Read the model definition and answer for the solid it produces. Units are mm, in the model's axes. Face numbers are marked on the shaded views. A direction names the side the tool comes from. Give positions to 0.01 mm unless a question says otherwise; leave off trailing zeros. Order: outer loops, then holes, each group sorted by start corner. A loop starts at its lowest first (then second) coordinate and runs counter-clockwise, first axis right, second up. Notation, with made-up numbers: (-33, 10) - (-26, 10) arc R32 ccw to (-26, 37) - close; hole circle Ø10 at (-8, -10.75). An arc over 180 degrees is marked (long way). Use a Markdown table: item, result. Add a question column.
1. A cutting plane is placed at D-D on x = 7.5. Determine the outline of the cut face in (y, z).
2. A flat-ended cylindrical pin translates along its axis: P1, Ø1.5, axis at x = -20.5, y = 2.5, coming from the +Z side. Find the tip coordinate at first contact, or state that the pin passes through.
3. A cutting plane is placed at C-C on z = 7.75. Determine the outline of the cut face in (x, y).
4. A cutting plane is placed at A-A on y = 0. Determine the outline of the cut face in (x, z).
5. Which of the six approach directions +Z, -Z, +X, -X, +Y, -Y give full straight-line access (tool end or side, diameter ignored) to the marked faces 1, 2 and 3?
6. A cutting plane is placed at B-B on y = -24.5. Determine the outline of the cut face in (x, z).
7. Consider L1, parallel to X at y = 0, z = 1.5; L2, parallel to X at y = -11, z = 3.75; L3, parallel to Y at x = -2, z = 3.5. Determine where each line is inside the solid, lowest interval first.
8. For a pull along Y with two mould halves and no side action, classify the marked faces 4, 5 and 6 as released by +Y, released by -Y, zero draft, split by the parting line, or undercut.
```python
from build123d import *

# Parameters (mm, degrees)
F0_W     = 56.9
F0_H     = 61.77927
F0_R     = 4.45
F1_DEPTH = 3
F2_R     = 4.45
F4_DEPTH = 10
F5_DEPTH = 3
F6_R     = 1.25
F7_DEPTH = 40


with BuildPart() as f1:
    # F0 (on Top) → F1 (new body)
    with BuildSketch(Plane.XY):
        Rectangle(F0_W, F0_H)
        with BuildLine():
            Line((1.5, -16.92031), (1.5, -26.92031))
            ThreePointArc((1.5, -26.92031), (1.06066, -27.98097), (0, -28.42031))
            ThreePointArc((0, -28.42031), (-1.06066, -27.98097), (-1.5, -26.92031))
            Line((-1.5, -26.92031), (-1.5, -16.92031))
            ThreePointArc((-1.5, -16.92031), (-1.06066, -15.85965), (0, -15.42031))
            ThreePointArc((0, -15.42031), (1.06066, -15.85965), (1.5, -16.92031))
        make_face(mode=Mode.SUBTRACT)
        with BuildLine():
            Line((-23.42031, -3.5), (-23.42031, 0))
            Line((-23.42031, 0), (-23.42031, 3.5))
            ThreePointArc((-23.42031, 3.5), (-21.92031, 5), (-20.42031, 3.5))
            Line((-20.42031, 3.5), (-20.42031, 0))
            Line((-20.42031, 0), (-20.42031, -3.5))
            ThreePointArc((-20.42031, -3.5), (-21.92031, -5), (-23.42031, -3.5))
        make_face(mode=Mode.SUBTRACT)
        with Locations((-20, 12)):
            Circle(F0_R, mode=Mode.SUBTRACT)
        with BuildLine():
            Line((-11.5, -3.5), (-11.5, 0))
            Line((-11.5, 0), (-11.5, 3.5))
            ThreePointArc((-11.5, 3.5), (-8.131728, 11.631728), (0, 15))
            ThreePointArc((0, 15), (8.131728, 11.631728), (11.5, 3.5))
            Line((11.5, 3.5), (11.5, 0))
            Line((11.5, 0), (11.5, -3.5))
            ThreePointArc((11.5, -3.5), (8.131728, -11.631728), (0, -15))
            ThreePointArc((0, -15), (-8.131728, -11.631728), (-11.5, -3.5))
        make_face(mode=Mode.SUBTRACT)
        with BuildLine():
            Line((20.42031, -3.5), (20.42031, 0))
            Line((20.42031, 0), (20.42031, 3.5))
            ThreePointArc((20.42031, 3.5), (21.92031, 5), (23.42031, 3.5))
            Line((23.42031, 3.5), (23.42031, 0))
            Line((23.42031, 0), (23.42031, -3.5))
            ThreePointArc((23.42031, -3.5), (21.92031, -5), (20.42031, -3.5))
        make_face(mode=Mode.SUBTRACT)
        with Locations((20, 12)):
            Circle(F0_R, mode=Mode.SUBTRACT)
        with BuildLine():
            Line((-1.5, 16.92031), (-1.5, 26.92031))
            ThreePointArc((-1.5, 26.92031), (-1.06066, 27.98097), (0, 28.42031))
            ThreePointArc((0, 28.42031), (1.06066, 27.98097), (1.5, 26.92031))
            Line((1.5, 26.92031), (1.5, 16.92031))
            ThreePointArc((1.5, 16.92031), (1.06066, 15.85965), (0, 15.42031))
            ThreePointArc((0, 15.42031), (-1.06066, 15.85965), (-1.5, 16.92031))
        make_face(mode=Mode.SUBTRACT)
    extrude(amount=F1_DEPTH)

    # F2 (on face) → F4 (join)
    with BuildSketch(Plane.XY.offset(3)):
        with BuildLine():
            Line((-26.45, -30.889635), (-26.45, 9.411564))
            ThreePointArc((-26.45, 9.411564), (-13.05, 12), (-26.45, 14.588436))
            Line((-26.45, 14.588436), (-26.45, 28.889635))
            Line((-26.45, 28.889635), (26.45, 28.889635))
            Line((26.45, 28.889635), (26.45, 14.588436))
            ThreePointArc((26.45, 14.588436), (13.05, 12), (26.45, 9.411564))
            Line((26.45, 9.411564), (26.45, -30.889635))
            Line((26.45, -30.889635), (28.45, -30.889635))
            Line((28.45, -30.889635), (28.45, 30.889635))
            Line((28.45, 30.889635), (-28.45, 30.889635))
            Line((-28.45, 30.889635), (-28.45, -30.889635))
            Line((-28.45, -30.889635), (-26.45, -30.889635))
        make_face()
        with Locations((-20, 12)):
            Circle(F2_R, mode=Mode.SUBTRACT)
        with Locations((20, 12)):
            Circle(F2_R, mode=Mode.SUBTRACT)
    extrude(amount=F4_DEPTH)

    # F3 (on face) → F5 (join)
    with BuildSketch(Plane.XY.offset(3)):
        with BuildLine():
            ThreePointArc((-19.42031, 3.5), (-21.92031, 6), (-24.42031, 3.5))
            Line((-24.42031, 3.5), (-24.42031, -3.5))
            ThreePointArc((-24.42031, -3.5), (-21.92031, -6), (-19.42031, -3.5))
            Line((-19.42031, -3.5), (-19.42031, 3.5))
        make_face()
        with BuildLine():
            ThreePointArc((-23.42031, 3.5), (-21.92031, 5), (-20.42031, 3.5))
            Line((-20.42031, 3.5), (-20.42031, -3.5))
            ThreePointArc((-20.42031, -3.5), (-21.92031, -5), (-23.42031, -3.5))
            Line((-23.42031, -3.5), (-23.42031, 3.5))
        make_face(mode=Mode.SUBTRACT)
        with BuildLine():
            Line((2.5, 16.92031), (2.5, 26.92031))
            ThreePointArc((2.5, 26.92031), (0, 29.42031), (-2.5, 26.92031))
            Line((-2.5, 26.92031), (-2.5, 16.92031))
            Line((-2.5, 16.92031), (-2.5, 14.724972))
            ThreePointArc((-2.5, 14.724972), (0, 15), (2.5, 14.724972))
            Line((2.5, 14.724972), (2.5, 16.92031))
        make_face()
        with BuildLine():
            Line((-1.5, 16.92031), (-1.5, 26.92031))
            ThreePointArc((-1.5, 26.92031), (0, 28.42031), (1.5, 26.92031))
            Line((1.5, 26.92031), (1.5, 16.92031))
            ThreePointArc((1.5, 16.92031), (0, 15.42031), (-1.5, 16.92031))
        make_face(mode=Mode.SUBTRACT)
        with BuildLine():
            Line((24.42031, -3.5), (24.42031, 3.5))
            ThreePointArc((24.42031, 3.5), (21.92031, 6), (19.42031, 3.5))
            Line((19.42031, 3.5), (19.42031, -3.5))
            ThreePointArc((19.42031, -3.5), (21.92031, -6), (24.42031, -3.5))
        make_face()
        with BuildLine():
            ThreePointArc((20.42031, 3.5), (21.92031, 5), (23.42031, 3.5))
            Line((23.42031, 3.5), (23.42031, -3.5))
            ThreePointArc((23.42031, -3.5), (21.92031, -5), (20.42031, -3.5))
            Line((20.42031, -3.5), (20.42031, 3.5))
        make_face(mode=Mode.SUBTRACT)
        with BuildLine():
            ThreePointArc((-2.5, -26.92031), (0, -29.42031), (2.5, -26.92031))
            Line((2.5, -26.92031), (2.5, -16.92031))
            Line((2.5, -16.92031), (2.5, -14.724972))
            ThreePointArc((2.5, -14.724972), (0, -15), (-2.5, -14.724972))
            Line((-2.5, -14.724972), (-2.5, -16.92031))
            Line((-2.5, -16.92031), (-2.5, -26.92031))
        make_face()
        with BuildLine():
            Line((1.5, -16.92031), (1.5, -26.92031))
            ThreePointArc((1.5, -26.92031), (0, -28.42031), (-1.5, -26.92031))
            Line((-1.5, -26.92031), (-1.5, -16.92031))
            ThreePointArc((-1.5, -16.92031), (0, -15.42031), (1.5, -16.92031))
        make_face(mode=Mode.SUBTRACT)
    extrude(amount=F5_DEPTH)

    # F6 (on face) → F7 (cut)
    with BuildSketch(Plane.XZ.offset(30.889635)):
        with Locations((-20, 10)):
            Circle(F6_R)
        with Locations((20, 10)):
            Circle(F6_R)
    extrude(amount=-F7_DEPTH, mode=Mode.SUBTRACT)


solid = f1.part
```
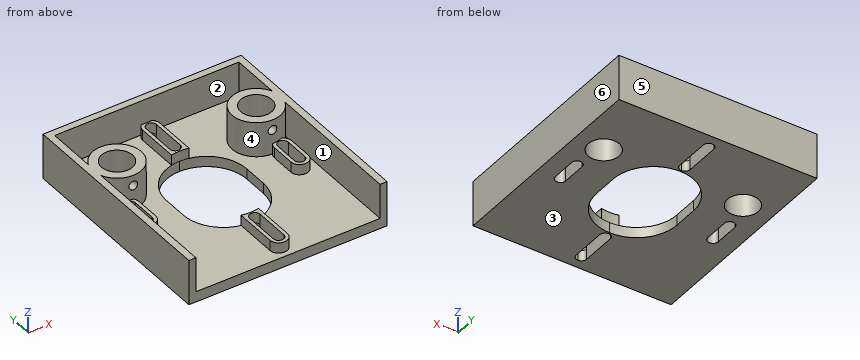
Output values:
| question | item | result |
|---|---|---|
| 1 | outline | (-30.89, 0) - (-12.22, 0) - (-12.22, 3) - (-30.89, 3) - close; (12.22, 0) - (30.89, 0) - (30.89, 13) - (28.89, 13) - (28.89, 3) - (12.22, 3) - close |
| 2 | P1 | z = 6 |
| 3 | outline | (-28.45, -30.89) - (-26.45, -30.89) - (-26.45, 9.41) arc R6.95 ccw (long way) to (-26.45, 14.59) - (-26.45, 28.89) - (26.45, 28.89) - (26.45, 14.59) arc R6.95 ccw (long way) to (26.45, 9.41) - (26.45, -30.89) - (28.45, -30.89) - (28.45, 30.89) - (-28.45, 30.89) - close; hole circle Ø8.9 at (-20, 12); hole circle Ø8.9 at (20, 12) |
| 4 | outline | (-28.45, 0) - (-23.42, 0) - (-23.42, 6) - (-24.42, 6) - (-24.42, 3) - (-26.45, 3) - (-26.45, 13) - (-28.45, 13) - close; (-20.42, 0) - (-11.5, 0) - (-11.5, 3) - (-19.42, 3) - (-19.42, 6) - (-20.42, 6) - close; (11.5, 0) - (20.42, 0) - (20.42, 6) - (19.42, 6) - (19.42, 3) - (11.5, 3) - close; (23.42, 0) - (28.45, 0) - (28.45, 13) - (26.45, 13) - (26.45, 3) - (24.42, 3) - (24.42, 6) - (23.42, 6) - close |
| 5 | face 1 | +Z, -Y |
| 5 | face 2 | +Z |
| 5 | face 3 | -Z, +X, -X, +Y, -Y |
| 6 | outline | (-28.45, 0) - (-1.5, 0) - (-1.5, 6) - (-2.5, 6) - (-2.5, 3) - (-26.45, 3) - (-26.45, 13) - (-28.45, 13) - close; (1.5, 0) - (28.45, 0) - (28.45, 13) - (26.45, 13) - (26.45, 3) - (2.5, 3) - (2.5, 6) - (1.5, 6) - close |
| 7 | L1 | -28.45 to -23.42, -20.42 to -11.5, 11.5 to 20.42, 23.42 to 28.45 |
| 7 | L2 | -28.45 to -26.45, 26.45 to 28.45 |
| 7 | L3 | -28.42 to -14.82, 14.82 to 28.42, 28.89 to 30.89 |
| 8 | face 4 | undercut |
| 8 | face 5 | released by +Y |
| 8 | face 6 | zero draft |
